Part print with two shaded views. Sizes in mm from the minimum x, y, z corner. A direction names the side the tool comes from. Give positions to 0.01 mm unless a question says otherwise; leave off trailing zeros. Write each loop counter-clockwise with the first axis right and the second up, starting at its lowest first coordinate (ties: lowest second). Pieces come first, ordered by that corner, then holes.
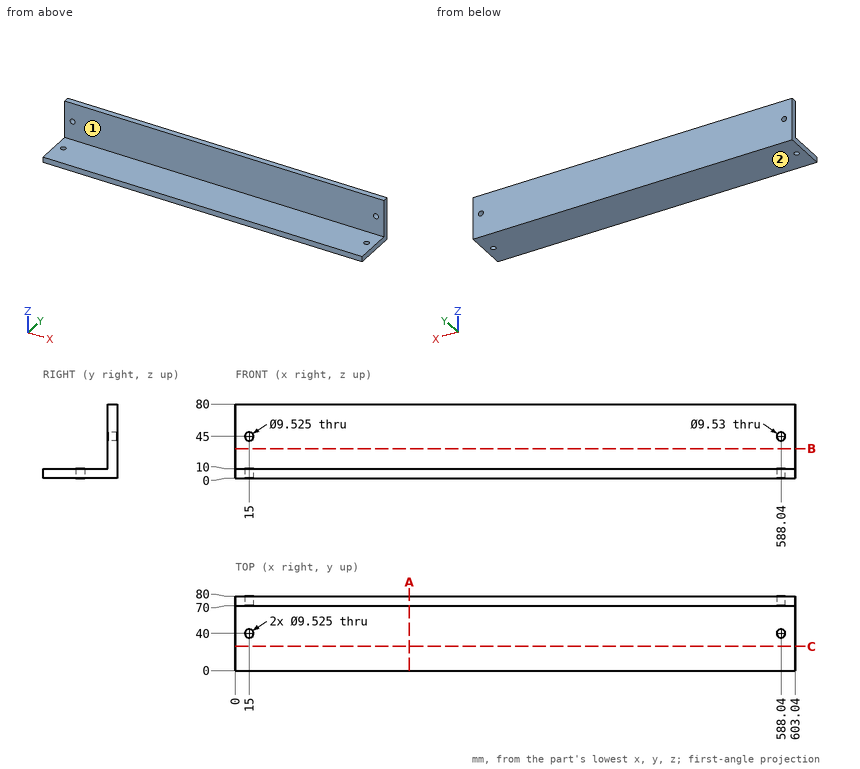
(1) Probe line 1 (Z direction, x = 15, y = 78); line 2 (Y direction, x = 15, z = 4.75); line 3 (Y direction, x = 80.5, z = 23). List the from-to ranges inside material, lowest first.
(2) Drop a flat-ended pin along its axis: pin 1 (15 mm diameter, centred on x = 15, y = 40, fed in from +Z). Give the stop position or say it passes through.
(3) Saw through at A-A, the plane x = 187.5. List the corners of the cut face in (y, z), plus the area to 3 significant figures.
(4) 3-axis set-ups, long thin cutter, end or side, ignore diameter. For the marked faces 1 and 2: which of +Z, -Z, +X, -X, +Y, -Y reach the whole face in a straight line?
(5) Saw through at C-C, the plane y = 26. List the corners of the cut face in (x, z), plus the area to 3 significant figures.
(6) Saw through at B-B, the plane z = 32. List the corners of the cut face in (x, y).
Computed values:
1. line 1: z = 0 to 40.24, 49.76 to 80
1. line 2: y = 0 to 35.24, 44.76 to 80
1. line 3: y = 70 to 80
2. pin 1: stops at z = 10
3. outline: (0, 0) - (80, 0) - (80, 80) - (70, 80) - (70, 10) - (0, 10) - close
3. area: 1,500 mm2
4. face 1: +Z, +X, -X, -Y
4. face 2: -Z, +X, -X, +Y, -Y
5. outline: (0, 0) - (603.04, 0) - (603.04, 10) - (0, 10) - close
5. area: 6,030 mm2
6. outline: (0, 70) - (603.04, 70) - (603.04, 80) - (0, 80) - close
